from build123d import *

# Parameters (mm, degrees)
SKETCH_1_R          = 52
SKETCH_1_R_2        = 1.55
SKETCH_1_R_3        = 40
EXTRUDE_1_DEPTH     = 3
EXTRUDE_START       = -3
SKETCH_2_R          = 40
SKETCH_2_R_2        = 24
EXTRUDE_2_DEPTH     = 3
CUT_EXTRUDE_1_DEPTH = 10
SKETCH_5_R          = 63.024090269
SKETCH_5_R_2        = 50
CUT_EXTRUDE_2_DEPTH = 10


with BuildPart() as part:
    # 草图1 → 凸台-拉伸1 (new body)
    with BuildSketch(Plane.XY):
        Circle(SKETCH_1_R)
        with Locations((46, 0)):
            Circle(SKETCH_1_R_2, mode=Mode.SUBTRACT)
        with Locations((23, -39.837168574)):
            Circle(SKETCH_1_R_2, mode=Mode.SUBTRACT)
        with Locations((-23, -39.837168574)):
            Circle(SKETCH_1_R_2, mode=Mode.SUBTRACT)
        with Locations((-46, 0)):
            Circle(SKETCH_1_R_2, mode=Mode.SUBTRACT)
        with Locations((-23, 39.837168574)):
            Circle(SKETCH_1_R_2, mode=Mode.SUBTRACT)
        with Locations((23, 39.837168574)):
            Circle(SKETCH_1_R_2, mode=Mode.SUBTRACT)
        Circle(SKETCH_1_R_3, mode=Mode.SUBTRACT)
    extrude(amount=EXTRUDE_1_DEPTH)

    # 草图2 → 凸台-拉伸2 (add)
    with BuildSketch(Plane.XY.offset(3).offset(EXTRUDE_START)):
        Circle(SKETCH_2_R)
        Circle(SKETCH_2_R_2, mode=Mode.SUBTRACT)
    extrude(amount=EXTRUDE_2_DEPTH)

    # 草图4 → 切除-拉伸1 (cut)
    with BuildSketch(Plane(origin=(0, 0, 0), x_dir=(-1, 0, 0), z_dir=(0, 0, -1))):
        with BuildLine():
            ThreePointArc((38.356187762, 13.472205401), (20.326690938, 35.206861455), (-7.510821758, 39.953535695))
            ThreePointArc((-7.510821758, 39.953535695), (-11.224371039, 34.520536752), (-5.791372097, 30.806987471))
            ThreePointArc((-5.791372097, 30.806987471), (15.673309062, 27.146967618), (29.575319812, 10.388018377))
            ThreePointArc((29.575319812, 10.388018377), (35.507847299, 7.539677914), (38.356187762, 13.472205401))
        make_face()
        with BuildLine():
            ThreePointArc((-5.791372097, -30.806987471), (15.673309062, -27.146967618), (29.575319812, -10.388018377))
            ThreePointArc((29.575319812, -10.388018377), (35.507847299, -7.539677914), (38.356187762, -13.472205401))
            ThreePointArc((38.356187762, -13.472205401), (20.326690938, -35.206861455), (-7.510821758, -39.953535695))
            ThreePointArc((-7.510821758, -39.953535695), (-11.224371039, -34.520536752), (-5.791372097, -30.806987471))
        make_face()
        with BuildLine():
            ThreePointArc((-23.783947715, 20.418969094), (-31.346618124, 0), (-23.783947715, -20.418969094))
            ThreePointArc((-23.783947715, -20.418969094), (-24.28347626, -26.980858838), (-30.845366003, -26.481330293))
            ThreePointArc((-30.845366003, -26.481330293), (-40.653381876, 0), (-30.845366003, 26.481330293))
            ThreePointArc((-30.845366003, 26.481330293), (-24.28347626, 26.980858838), (-23.783947715, 20.418969094))
        make_face()
    extrude(amount=-CUT_EXTRUDE_1_DEPTH, mode=Mode.SUBTRACT)

    # 草图5 → 切除-拉伸2 (cut)
    with BuildSketch(Plane(origin=(0, 0, 0), x_dir=(-1, 0, 0), z_dir=(0, 0, -1))):
        Circle(SKETCH_5_R)
        Circle(SKETCH_5_R_2, mode=Mode.SUBTRACT)
    extrude(amount=-CUT_EXTRUDE_2_DEPTH, mode=Mode.SUBTRACT)


solid = part.part
Source: CAD feature listing. Evaluate the final solid. Frame: model axes, mm. A direction names the side the tool comes from. Give positions to 0.01 mm unless a question says otherwise; leave off trailing zeros. Write each loop counter-clockwise with the first axis right and the second up, starting at its lowest first coordinate (ties: lowest second). Pieces come first, ordered by that corner, then holes. Notation, with made-up numbers: (-10, -36) -> (48, -36) arc R16 ccw to (48, -26) -> close; hole circle Ø3 at (-25, 38). An arc over 180 degrees is marked (long way). Write item = value, one per line.
Q1. Mould query, pull axis X, two halves, no side actions, for faces 1 (the face through (22, 12, 3)), 2 (the face through (-47.69, 15.02, 1.48)), 3 (the face through (11.24, 34.62, 1.48)). Classes: +X half, -X half, draft (parallel to the pull), parting line (faces both ways), or undercut.
Here are the results:
face_1 = draft
face_2 = parting line
face_3 = undercut
Q2. Cut plane C-C on y = 33.5. Return loops of the section in (x, z), then the cut area to 3 significant figures.
Here are the results:
outline = (-37.12, 0) -> (-23.03, 0) -> (-23.03, 3) -> (-37.12, 3) -> close; (10.91, 0) -> (37.12, 0) -> (37.12, 3) -> (10.91, 3) -> close
area = 121 mm²
Q3. Line query: line 1 (X direction, y = 26.5, z = 1.85); line 2 (Y direction, x = -37, z = 2); line 3 (Y direction, x = -34.5, z = 2.35). Output: solid intervals per line, ascending. Write a range as from..to.
Here are the results:
line_1 = -42.4..-30.83, -16.74..23.8, 30.83..42.4
line_2 = -33.63..-16.84, -8.4..8.4, 16.84..33.63
line_3 = -36.19..-21.5, -7.31..7.31, 21.5..36.19
Q4. Cut plane A-A on y = 0. Return loops of the section in (x, z).
Here are the results:
outline = (-50, 0) -> (-47.55, 0) -> (-47.55, 3) -> (-50, 3) -> close; (-44.45, 0) -> (-24, 0) -> (-24, 3) -> (-44.45, 3) -> close; (24, 0) -> (31.35, 0) -> (31.35, 3) -> (24, 3) -> close; (40.65, 0) -> (44.45, 0) -> (44.45, 3) -> (40.65, 3) -> close; (47.55, 0) -> (50, 0) -> (50, 3) -> (47.55, 3) -> close
Q5. Cut plane B-B on x = 0. Return loops of the section in (y, z), then the cut area to 3 significant figures.
Here are the results:
outline = (-50, 0) -> (-40.65, 0) -> (-40.65, 3) -> (-50, 3) -> close; (-31.35, 0) -> (-24, 0) -> (-24, 3) -> (-31.35, 3) -> close; (24, 0) -> (31.35, 0) -> (31.35, 3) -> (24, 3) -> close; (40.65, 0) -> (50, 0) -> (50, 3) -> (40.65, 3) -> close
area = 100 mm²
Q6. Reachability of faces 4 (the face through (22, 12, 0)), 5 (the face through (-20.68, -35, 1.48)) from +Z, -Z, +X, -X, +Y, -Y: full face, straight path, thin tool, end or side. Return the list, or none.
Here are the results:
face_4 = -Z, +X, -X, +Y, -Y
face_5 = +Z, -Z
Q7. Cut plane D-D on z = 2.1. State how many separate pieces and enclosed holes the cut face has, then the cut area to 3 significant figures.
Here are the results:
separate_pieces = 1
enclosed_holes = 10
area = 4,370 mm²
